The drawing under review shows one solid part. Ordinate dimensions are in mm from its lowest x, y, z. Round coordinates to 2 decimals unless told otherwise and drop trailing zeros. Write each loop counter-clockwise with the first axis right and the second up, starting at its lowest first coordinate (ties: lowest second). Pieces come first, ordered by that corner, then holes.
Item 1: Add section B-B (z = 30). Give the boundary of the cut face in (x, y).
Item 2: Add section D-D (z = 5.5). Give the boundary of the cut face in (x, y).
Item 3: Add section A-A (x = 10). Give the boundary of the cut face in (y, z).
Item 4: Draft analysis for pull direction X (two halves, no side actions). For the marked faces 1, 2 and 3, state which applies: +X half, -X half, draft (parallel to the pull), parting line (faces both ways), or undercut.
Item 5: Clearance check with flat-ended pins moving along their axes: pin 1 Ø5 at (x, y) = (12, 6) entering from -Z; pin 2 Ø4 at (x, y) = (10, 7.5) entering from -Z. State where each tip first meets the part, or that it passes through.
Item 6: Add section C-C (y = 7.5). Give the boundary of the cut face in (x, z), plus the area to 3 significant figures.
Item 7: To check wall thickness, follow L1, parallel to X at y = 3.5, z = 30; L2, parallel to Z at x = 10.25, y = 6; L3, parallel to Y at x = 10, z = 9.5. State the ranges of each line that lie inside material, in increasing order.
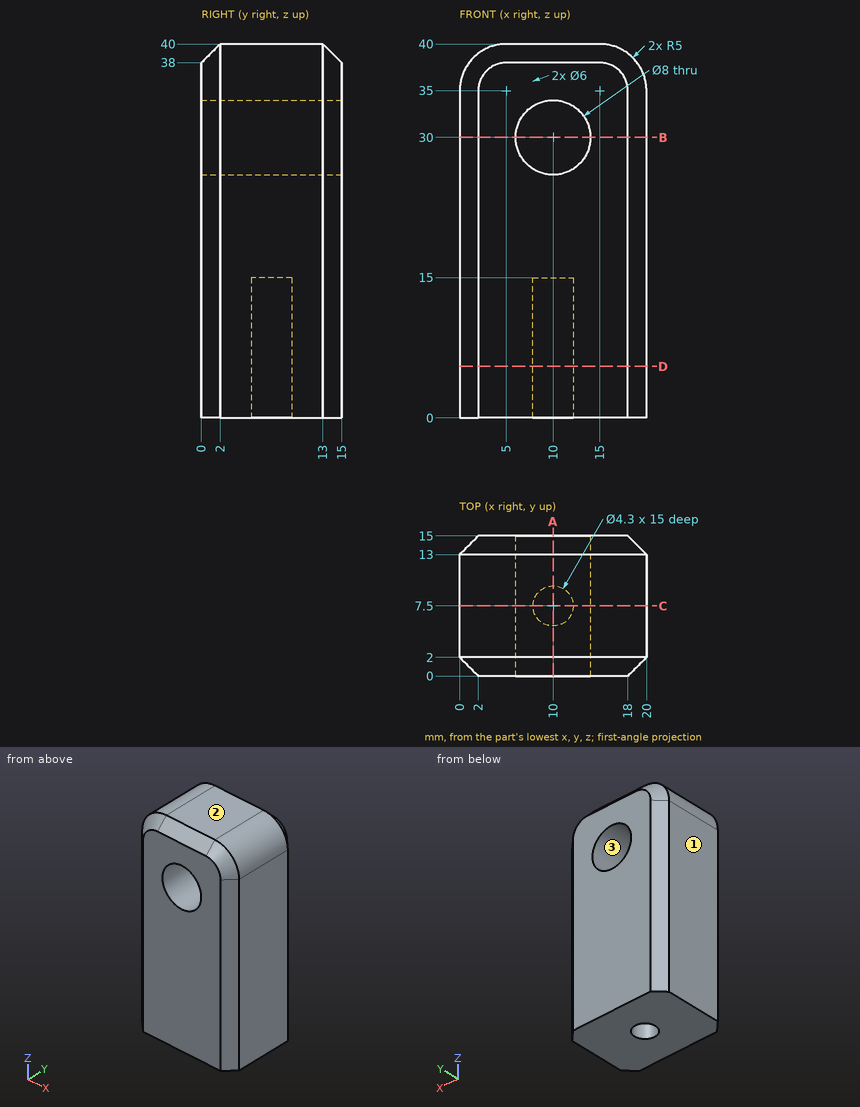
Numbers:
1. outline: (0, 2) - (2, 0) - (6, 0) - (6, 15) - (2, 15) - (0, 13) - close; (14, 0) - (18, 0) - (20, 2) - (20, 13) - (18, 15) - (14, 15) - close
2. outline: (0, 2) - (2, 0) - (18, 0) - (20, 2) - (20, 13) - (18, 15) - (2, 15) - (0, 13) - close; hole circle Ø4.3 at (10, 7.5)
3. outline: (0, 0) - (5.35, 0) - (5.35, 15) - (9.65, 15) - (9.65, 0) - (15, 0) - (15, 26) - (0, 26) - close; (0, 34) - (15, 34) - (15, 38) - (13, 40) - (2, 40) - (0, 38) - close
4. face 1: -X half
4. face 2: draft
4. face 3: undercut
5. pin 1: stops at z = 0
5. pin 2: stops at z = 15
6. outline: (0, 0) - (7.85, 0) - (7.85, 15) - (12.15, 15) - (12.15, 0) - (20, 0) - (20, 35) arc R5 ccw to (15, 40) - (5, 40) arc R5 ccw to (0, 35) - close; hole circle Ø8 at (10, 30)
6. area: 675 mm2
7. L1: x = 0 to 6, 14 to 20
7. L2: z = 15 to 26.01, 33.99 to 40
7. L3: y = 0 to 5.35, 9.65 to 15
